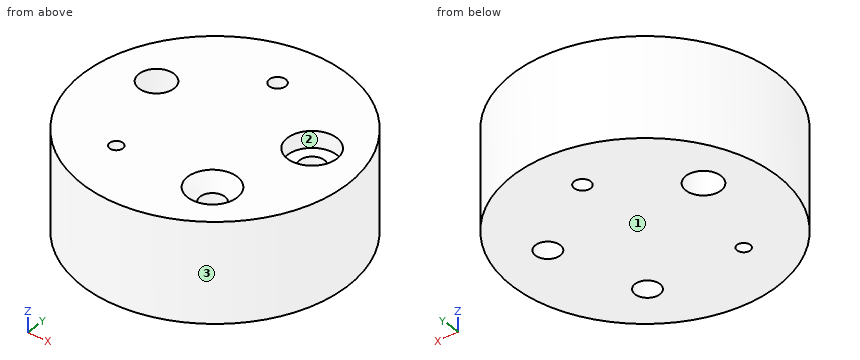
```python
from build123d import *

# Parameters (mm, degrees)
F0_R           = 50.8
F1_DEPTH       = 38.1
F3_D           = 6.35
F4_D           = 9.525
F4_CBORE_D     = 19.05
F4_CBORE_DEPTH = 6.35
F5_D           = 9.525
F5_CSINK_D     = 19.05
F5_CSINK_ANGLE = 82
F6_D           = 5.1054
F7_D           = 13.49248


with BuildPart() as f1:
    # F0 (on Top) → F1 (new body)
    with BuildSketch(Plane.XY):
        Circle(F0_R)
    extrude(amount=F1_DEPTH)

    # F3 (through all)
    with Locations(Plane.XY.offset(38.1)):
        with Locations((0, 31.75)):
            Hole(F3_D / 2)

    # F4 (through all)
    with Locations(Plane.XY.offset(38.1)):
        with Locations((30.1960443924, 9.8112895714)):
            CounterBoreHole(F4_D / 2, F4_CBORE_D / 2, F4_CBORE_DEPTH)

    # F5 (through all)
    with Locations(Plane.XY.offset(38.1)):
        with Locations((18.6621817603, -25.6862895714)):
            CounterSinkHole(F5_D / 2, F5_CSINK_D / 2, counter_sink_angle=F5_CSINK_ANGLE)

    # F6 (through all)
    with Locations(Plane.XY.offset(38.1)):
        with Locations((-18.6621817603, -25.6862895714)):
            Hole(F6_D / 2)

    # F7 (through all)
    with Locations(Plane.XY.offset(38.1)):
        with Locations((-30.1960443924, 9.8112895714)):
            Hole(F7_D / 2)


solid = f1.part
```
For this review, take the finished solid that the model builds, in its own axes (mm). Face numbers are marked on the shaded views. Give positions to 0.01 mm unless a question says otherwise; leave off trailing zeros. Write each loop counter-clockwise with the first axis right and the second up, starting at its lowest first coordinate (ties: lowest second). Pieces come first, ordered by that corner, then holes.
Item 1: Take a section at C-C (z = 14.5). Give the number of separate pieces and of enclosed holes in the cut face, and give its area (3 significant figures).
Item 2: Insertion check: P1, Ø6, axis at x = -18.66, y = -25.69, coming from the +Z side; P2, Ø1.5, axis at y = 28, z = 34, coming from the -X side; P3, Ø8, axis at x = -35, z = 25.5, coming from the -Y side; P4, Ø17, axis at x = 30.2, y = 9.81, coming from the +Z side. Each pin has a flat end and moves straight along its axis. Give the tip position at first contact, or say it passes through.
Item 3: Wall thickness on probe 1 along X at (y, z) = (12, 12); probe 2 along X at (y, z) = (10, 27.5); probe 3 along X at (y, z) = (0.5, 30): over which ranges is each line inside the solid? List them lowest first.
Item 4: Take a section at D-D (x = -39). Give the boundary of the cut face in (y, z), and give its area (3 significant figures).
Item 5: The part is to be moulded in two halves that separate along X. For the marked faces 1, 2 and 3, say which applies: +X half, -X half, draft (parallel to the pull), parting line (faces both ways), or undercut.
Item 6: Take a section at B-B (y = 31.75). Give the boundary of the cut face in (x, z) (3 decimals), and give its area (3 significant figures).
Item 7: Take a section at A-A (x = 0). Give the boundary of the cut face in (y, z) (3 decimals).
Established:
1. separate pieces: 1
1. enclosed holes: 5
1. area: 7,770 mm2
2. P1: stops at z = 38.1
2. P2: stops at x = -42.87
2. P3: stops at y = -40.24
2. P4: stops at z = 31.75
3. probe 1: x = -49.36 to -36.58, -23.81 to 25.97, 34.43 to 49.36
3. probe 2: x = -49.81 to -36.94, -23.45 to 25.44, 34.95 to 49.81
3. probe 3: x = -50.8 to 50.8
4. outline: (-32.55, 0) - (32.55, 0) - (32.55, 38.1) - (-32.55, 38.1) - close
4. area: 2,480 mm2
5. face 1: draft
5. face 2: undercut
5. face 3: parting line
6. outline: (-39.656, 0) - (-3.175, 0) - (-3.175, 38.1) - (-39.656, 38.1) - close; (3.175, 0) - (39.656, 0) - (39.656, 38.1) - (3.175, 38.1) - close
6. area: 2,780 mm2
7. outline: (-50.8, 0) - (28.575, 0) - (28.575, 38.1) - (-50.8, 38.1) - close; (34.925, 0) - (50.8, 0) - (50.8, 38.1) - (34.925, 38.1) - close
